Source: three-view drawing plus pictorial views. Frame: mm from the lowest corner of the part. Give positions to 0.01 mm unless a question says otherwise; leave off trailing zeros. Loops run counter-clockwise (first coordinate to the right, second up) from the corner with the lowest first, then second, coordinate; pieces in that order, holes last.
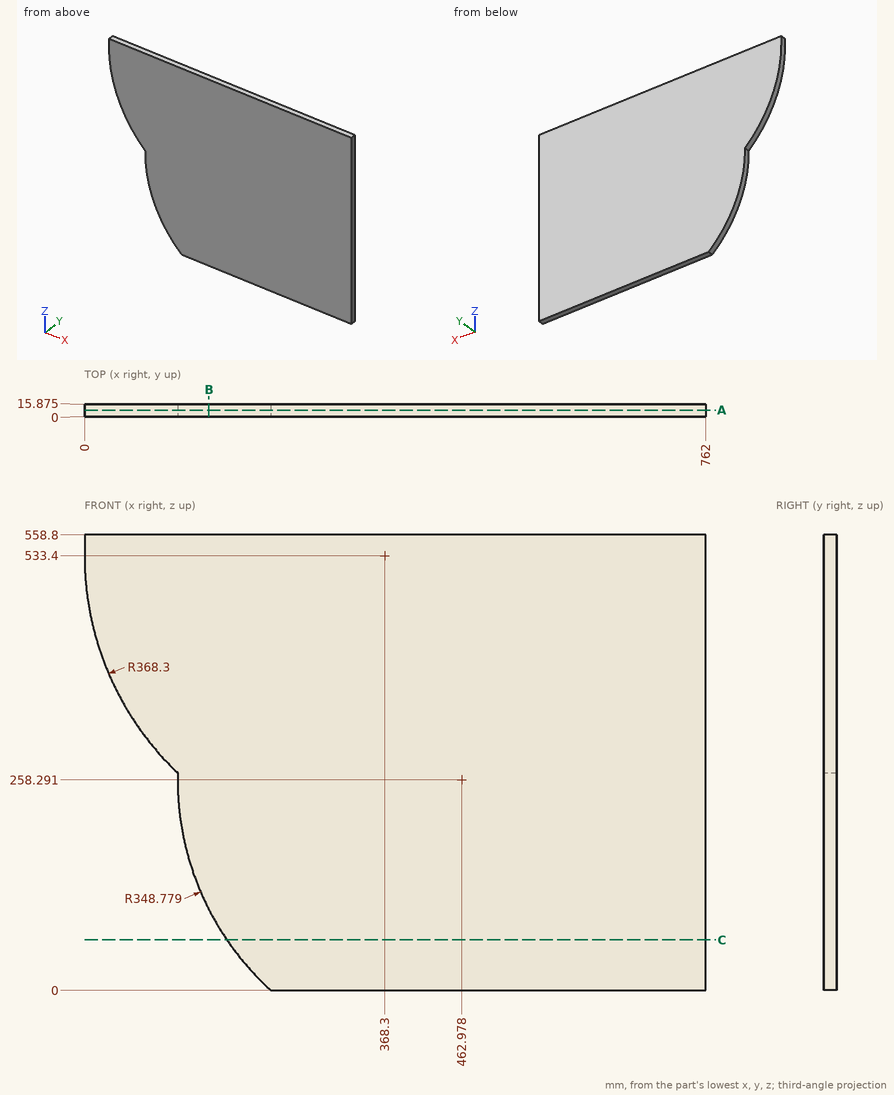
(1) Cut plane A-A (y = 8.5). Return the cut outline in (x, z), and give its area (3 significant figures).
Values follow:
outline: (0, 533.4) arc R368.3 ccw to (114.3, 266.7) arc R348.78 ccw to (228.6, 0) - (762, 0) - (762, 558.8) - (0, 558.8) - close
area: 377,000 mm2
(2) Ray query, probe 1 along X at (y, z) = (1.75, 530.5); probe 2 along X at (y, z) = (5.75, 250); probe 3 along Z at (x, y) = (89, 5) (1 decimal). Return the intervals inside material, ascending.
Values follow:
probe 1: x = 0.01 to 762
probe 2: x = 114.3 to 762
probe 3: z = 293.3 to 558.8
(3) Cut plane B-B (x = 152.5). Return the cut outline in (y, z) (1 decimal), and give its area (3 significant figures).
Values follow:
outline: (0, 99.4) - (15.9, 99.4) - (15.9, 558.8) - (0, 558.8) - close
area: 7,290 mm2
(4) Pin query (flat end, axial travel): pin 1 Ø3 at (y, z) = (3, 498.5) entering from -X; pin 2 Ø6 at (y, z) = (3, 268) entering from -X. Return the tip coordinate at first contact, or that it passes through.
Values follow:
pin 1: stops at x = 1.52
pin 2: stops at x = 109.86
(5) Cut plane C-C (z = 62). Return the cut outline in (x, y) (1 decimal), and give its area (3 significant figures).
Values follow:
outline: (174.7, 0) - (762, 0) - (762, 15.9) - (174.7, 15.9) - close
area: 9,320 mm2
